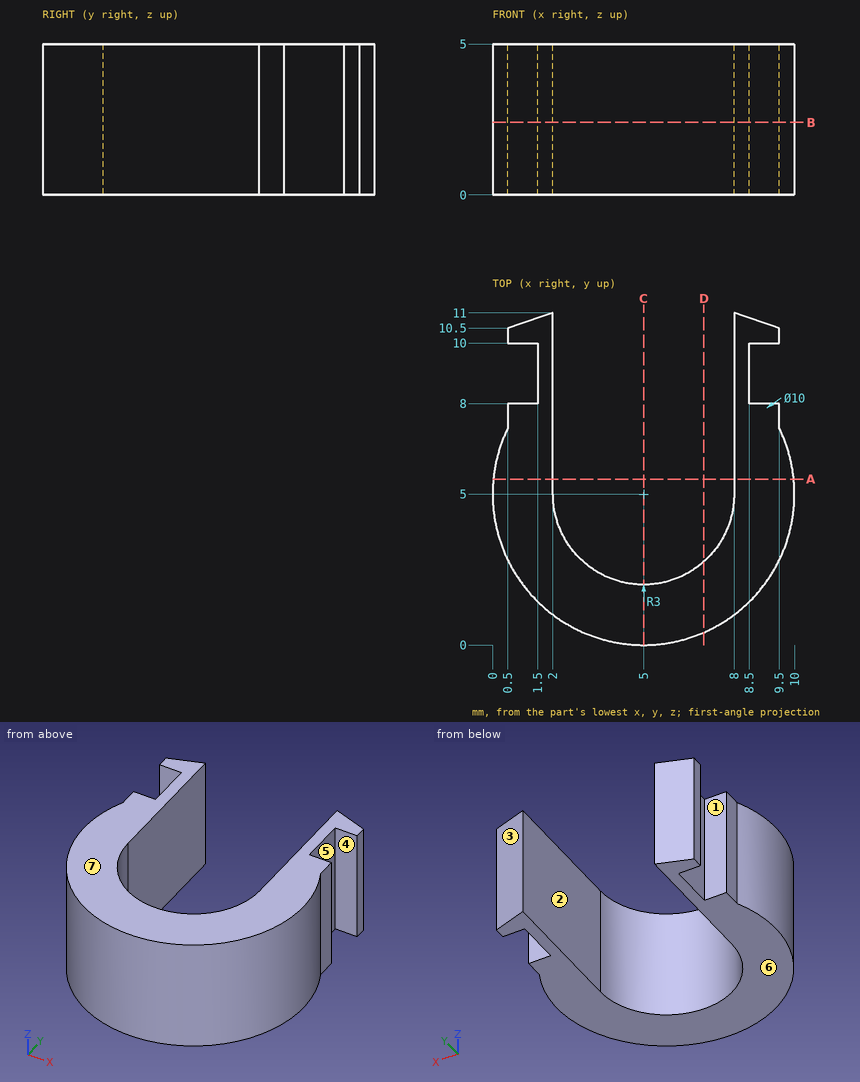
Here's the drawing with two shaded views (mm, measured from the low corner). I have some questions. A direction names the side the tool comes from. Round coordinates to 2 decimals unless told otherwise and drop trailing zeros. Loops run counter-clockwise (first coordinate to the right, second up) from the corner with the lowest first, then second, coordinate; pieces in that order, holes last. Notation, with made-up numbers: (38.5, -18.5) -> (46.5, -18.5) arc R11 ccw to (46.5, -14.5) -> close; hole circle Ø11 at (29.5, 20). An arc over 180 degrees is marked (long way). Answer as CSV lines item,"result". Start each with the question number.
1. Imagine slicing it at C-C on x = 5. Write out the boundary of the cut face in (y, z).
2. Imagine slicing it at A-A on y = 5.5. Write out the boundary of the cut face in (x, z), plus the area to 3 significant figures.
3. I'm going to push flat-ended pins straight in: P1, Ø0.9, axis at y = 7.5, z = 1.5, coming from the +X side; P2, Ø1, axis at x = 3, y = 4.5, coming from the +Z side; P3, Ø0.5, axis at x = 9, z = 3.5, coming from the +Y side; P4, Ø0.5, axis at x = 9, z = 3, coming from the -Y side. Where does each tip first touch, or does it pass through?
4. I need wall thicknesses on probe 1 along X at (y, z) = (9.25, 2.15); probe 2 along X at (y, z) = (7.25, 4.5); probe 3 along Y at (x, z) = (9.25, 1.05). Which ranges of each line are inside material? Lowest first, please. Write a range as from..to.
5. Imagine slicing it at B-B on z = 2.4. Write out the boundary of the cut face in (x, y).
6. For the marked faces 1, 2, 3 and 4, which set-ups out of +Z, -Z, +X, -X, +Y, -Y let a thin tool reach every point of the face, with its end or its side?
7. If we mould it in two halves opening along Z, with no side actions, what happens to the marked faces 5, 6 and 7? For each: pulls with the +Z half, pulls with the -Z half, needs draft (parallel to the pull), parting line crosses it, or undercut.
8. Imagine slicing it at D-D on x = 7. Write out the boundary of the cut face in (y, z), plus the area to 3 significant figures.
Solution:
1,outline,"(0, 0) -> (2, 0) -> (2, 5) -> (0, 5) -> close"
2,outline,"(0.03, 0) -> (2, 0) -> (2, 5) -> (0.03, 5) -> close; (8, 0) -> (9.97, 0) -> (9.97, 5) -> (8, 5) -> close"
2,area,"19.7 mm²"
3,P1,"x = 9.56"
3,P2,"through"
3,P3,"y = 10.75"
3,P4,"y = 1.69"
4,probe 1,"1.5..2, 8..8.5"
4,probe 2,"0.5..2, 8..9.5"
4,probe 3,"2.37..8, 10..10.58"
5,outline,"(0.5, 7.18) arc R5 ccw (long way) to (9.5, 7.18) -> (9.5, 8) -> (8.5, 8) -> (8.5, 10) -> (9.5, 10) -> (9.5, 10.5) -> (8, 11) -> (8, 5) arc R3 cw to (2, 5) -> (2, 11) -> (0.5, 10.5) -> (0.5, 10) -> (1.5, 10) -> (1.5, 8) -> (0.5, 8) -> close"
6,face 1,"+Z, -Z, -X"
6,face 2,"+Z, -Z, +Y"
6,face 3,"+Z, -Z, +X, +Y"
6,face 4,"+Z, -Z, +X"
7,face 5,"needs draft"
7,face 6,"pulls with the -Z half"
7,face 7,"pulls with the +Z half"
8,outline,"(0.42, 0) -> (2.76, 0) -> (2.76, 5) -> (0.42, 5) -> close"
8,area,"11.7 mm²"
